from build123d import *

# Parameters (mm, degrees)
F0_W     = 119.38
F0_H     = 100.33
F0_R     = 34.29
F1_DEPTH = 38.1
F4_DEPTH = 119.381
F5_R     = 5.08
F6_R     = 5.08
F7_R     = 5.08
F8_R     = 41.6341019148
F9_DEPTH = 36.83


with BuildPart() as f1:
    # F0 (on Front) → F1 (new body)
    with BuildSketch(Plane.XZ):
        with Locations((0, -3.175)):
            Rectangle(F0_W, F0_H)
        Circle(F0_R, mode=Mode.SUBTRACT)
    extrude(amount=-F1_DEPTH)

    # F3 (on face) → F4 (cut, through all)
    with BuildSketch(Plane.YZ.offset(59.69)):
        Polygon((28.9814, 7.6699430424), (0, 41.6043430424), (0, -53.34), (23.6982, -53.34), align=None)
    extrude(amount=-F4_DEPTH, mode=Mode.SUBTRACT)

    # F5
    f5_edges = [f1.edges().sort_by_distance(p)[0] for p in [
        (46.555596, 28.9814, 7.669943),
        (-46.555596, 28.9814, 7.669943),
    ]]
    fillet(f5_edges, radius=F5_R)

    # F6
    f6_edges = [f1.edges().sort_by_distance(p)[0] for p in [
        (0, 38.1, -53.34),
        (0, 23.6982, -53.34),
        (59.69, 30.8991, -53.34),
        (-59.69, 30.8991, -53.34),
    ]]
    fillet(f6_edges, radius=F6_R)

    # F7
    f7_edges = [f1.edges().sort_by_distance(p)[0] for p in [
        (0, 38.1, 46.99),
    ]]
    fillet(f7_edges, radius=F7_R)

    # F8 (on Front) → F9 (cut)
    with BuildSketch(Plane.XZ):
        Circle(F8_R)
    extrude(amount=-F9_DEPTH, mode=Mode.SUBTRACT)


solid = f1.part
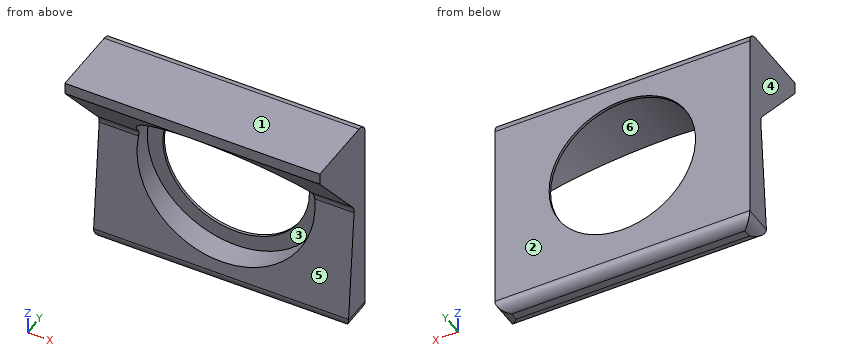
Can you work these out from the model? Positions are in its coordinate system, mm. Face numbers are marked on the shaded views. A direction names the side the tool comes from. Give positions to 0.01 mm unless a question says otherwise; leave off trailing zeros. Order: outer loops, then holes, each group sorted by start corner. A loop starts at its lowest first (then second) coordinate and runs counter-clockwise, first axis right, second up. Notation, with made-up numbers: M 31.5,54 L 48.5,54 A10 ccw 48.5,64 Z; hole C 75.25,-27 d9. An arc over 180 degrees is marked long. One line per question, with ' | ' between items.
Item 1: I'm going to push a flat-ended pin straight in: pin 1 Ø1.5 at (x, y) = (-44.5, 28.5) entering from -Z. Where does the tip first touch, or does it pass through?
Answer block:
pin 1: stops at z = -53.34
Item 2: Please list where these lines run through material, in increasing order: L1, parallel to Z at x = 0, y = 21; L2, parallel to Z at x = 0, y = 37; L3, parallel to X at y = 33, z = -38.
Answer block:
L1: z = 41.63 to 46.99 | L2: z = -51.42 to -34.29, 34.29 to 45.07 | L3: x = -59.69 to -17.01, 17.01 to 59.69
Item 3: Suppose I cut it at D-D, the plane z = 38. Write out the boundary of the cut face in (x, y), then the cut area to 3 significant figures.
Answer block:
outline: M -59.69,3.08 L -17.01,3.08 L -17.01,36.83 L 17.01,36.83 L 17.01,3.08 L 59.69,3.08 L 59.69,38.1 L -59.69,38.1 Z | area: 3,030 mm2
Item 4: Suppose I cut it at C-C, the plane z = -5. Write out the boundary of the cut face in (x, y), then the cut area to 3 significant figures.
Answer block:
outline: M -59.69,27.88 L -41.33,27.88 L -41.33,36.83 L -33.92,36.83 L -33.92,38.1 L -59.69,38.1 Z; M 33.92,36.83 L 41.33,36.83 L 41.33,27.88 L 59.69,27.88 L 59.69,38.1 L 33.92,38.1 Z | area: 394 mm2
Item 5: We'd pull the mould along Z, two halves only. Please class the marked faces 1, 2 and 3: released by +Z, released by -Z, zero draft, split by the parting line, or undercut.
Answer block:
face 1: released by +Z | face 2: zero draft | face 3: undercut
Item 6: Suppose I cut it at B-B, the plane x = -4.5. Write out the boundary of the cut face in (y, z).
Answer block:
outline: M 0,41.6 L 0.18,41.39 L 36.83,41.39 L 36.83,33.99 L 38.1,33.99 L 38.1,41.91 A5.08 ccw 33.02,46.99 L 0,46.99 Z; M 24.18,-47.82 A5.08 ccw 29.24,-53.34 L 33.02,-53.34 A5.08 ccw 38.1,-48.26 L 38.1,-33.99 L 36.83,-33.99 L 36.83,-41.39 L 24.73,-41.39 Z
Item 7: Suppose I cut it at A-A, the plane y = 31.5. Write out the boundary of the cut face in (x, z), then the cut area to 3 significant figures.
Answer block:
outline: M -59.69,-48.26 A5.08 ccw -54.61,-53.34 L 54.61,-53.34 A5.08 ccw 59.69,-48.26 L 59.69,46.99 L -59.69,46.99 Z; hole C 0,0 d83.27 | area: 6,520 mm2
Item 8: For the marked faces 4, 5 and 6, which set-ups out of +Z, -Z, +X, -X, +Y, -Y let a thin tool reach every point of the face, with its end or its side?
Answer block:
face 4: +Z, -Z, -X, +Y, -Y | face 5: +X, -X, -Y | face 6: -Y
